Autodesk Inventor part; units mm, degrees
ref_plane "YZ Plane" through (0, 0, 0) normal (1, 0, 0) x (0, 1, 0)
ref_plane "XZ Plane" through (0, 0, 0) normal (0, 1, 0) x (-1, 0, 0)
ref_plane "XY Plane" through (0, 0, 0) normal (0, 0, 1) x (1, 0, 0)
sketch "スケッチ1" plane through (0, 0, 0) normal (0, 0, 1) x (1, 0, 0)
  line L0 (0, 0) -> (15, 0)
  line L1 (15, 0) -> (15, 30)
  line L2 (15, 30) -> (0, 30)
  line L3 (0, 30) -> (0, 0)
  line L4 (1, 1) -> (14, 1)
  line L5 (14, 1) -> (14, 29)
  line L6 (14, 29) -> (1, 29)
  line L7 (1, 29) -> (1, 1)
  dimension "d0" = 15
  dimension "d1" = 30
  dimension "d2" = 13
  dimension "d3" = 28
  dimension "d4" = 1
  dimension "d5" = 1
extrude "押し出し1" add sketch "スケッチ1" along normal blind 330
sketch "スケッチ2" plane through (0, 30, 0) normal (0, 1, 0) x (1, 0, 0)
  circle A0 centre (7.5, -15) radius 1.6
  line L0 (0, 0) -> (0, -330)
  line L1 (15, 0) -> (0, 0)
  circle A1 centre (7.5, -25) radius 1.6
  circle A2 centre (7.5, -35) radius 1.6
  circle A3 centre (7.5, -315) radius 1.6
  line L2 (15, -330) -> (0, -330)
  circle A4 centre (7.5, -305) radius 1.6
  circle A5 centre (7.5, -295) radius 1.6
  dimension "d8" = 3.2
  dimension "d9" = 7.5
  dimension "d10" = 15
  dimension "d11" = 3.2
  dimension "d12" = 10
  dimension "d13" = 3.2
  dimension "d14" = 10
  dimension "d15" = 3.2
  dimension "d16" = 15
  dimension "d17" = 7.5
  dimension "d18" = 3.2
  dimension "d19" = 10
  dimension "d20" = 3.2
  dimension "d21" = 10
hole "穴1" at (7.5, 30, 315) at (7.5, 30, 305) at (7.5, 30, 295) at (7.5, 30, 15) at (7.5, 30, 25) at (7.5, 30, 35) direction (0, -1, 0) diameter 3.2 depth 30
sketch "スケッチ3" plane through (0, 0, 0) normal (-1, 0, 0) x (0, 0, 1)
  circle A0 centre (10, 15) radius 1.6
  line L0 (0, 0) -> (330, 0)
  line L1 (0, 30) -> (0, 0)
  circle A1 centre (20, 15) radius 1.6
  circle A2 centre (30, 15) radius 1.6
  circle A3 centre (320, 15) radius 1.6
  line L2 (330, 30) -> (330, 0)
  circle A4 centre (310, 15) radius 1.6
  circle A5 centre (300, 15) radius 1.6
  dimension "d29" = 3.2
  dimension "d30" = 15
  dimension "d31" = 10
  dimension "d32" = 3.2
  dimension "d33" = 3.2
  dimension "d34" = 10
  dimension "d35" = 10
  dimension "d36" = 3.2
  dimension "d37" = 15
  dimension "d38" = 10
  dimension "d39" = 3.2
  dimension "d40" = 3.2
  dimension "d41" = 10
  dimension "d42" = 10
  dimension "d43" = 15
  dimension "d44" = 15
  dimension "d45" = 15
  dimension "d46" = 15
hole "穴2" at (0, 15, 10) at (0, 15, 20) at (0, 15, 30) at (0, 15, 300) at (0, 15, 310) at (0, 15, 320) direction (1, 0, 0) diameter 3.2 depth 15
sketch "スケッチ4" plane through (0, 0, 0) normal (-1, 0, 0) x (0, 0, 1)
  line L0 (165, 29.8281) -> (165, -0.1719) construction
  line L1 (0, 1) -> (330, 1)
  line L2 (165, 29.8281) -> (195, 29.8281) construction
  line L3 (0, 30) -> (0, 0)
  dimension "d54" = 30
  dimension "d55" = 90
  dimension "d56" = 165
sketch "スケッチ5" plane through (0, 0, 0) normal (-1, 0, 0) x (0, 0, 1)
  point P0 (0, 0)
sketch "スケッチ6" plane through (0, 0, 0) normal (-1, 0, 0) x (0, 0, 1)
  circle A0 centre (205.5, 23) radius 1.6
  circle A1 centre (205.5, 7) radius 1.6
  line L0 (0, 30) -> (330, 30)
  line L1 (0, 0) -> (330, 0)
  line L2 (0, 30) -> (0, 0)
  circle A2 centre (268.95, 23) radius 1.6
  circle A3 centre (268.95, 7) radius 1.6
  dimension "d57" = 3.2
  dimension "d58" = 3.2
  dimension "d59" = 16
  dimension "d60" = 7
  dimension "d61" = 7
  dimension "d62" = 205.5
  dimension "d63" = 3.2
  dimension "d64" = 63.45
  dimension "d65" = 7
  dimension "d66" = 3.2
  dimension "d67" = 16
  dimension "d68" = 7
hole "穴3" at (0, 23, 205.5) at (0, 7, 205.5) at (0, 23, 268.95) at (0, 7, 268.95) direction (1, 0, 0) diameter 3.2 depth 15
equation "\"BendRadius\" = Thickness"
equation "\"BendReliefWidth\" = Thickness"
equation "\"BendReliefDepth\" = 0.5 * Thickness"
equation "\"CornerReliefSize\" = 4 * Thickness"
equation "\"MinimumRemnant\" = 2 * Thickness"
equation "\"TransitionRadius\" = BendRadius"
equation "\"JacobiRadiusSize\" = BendRadius"
equation "\"GapSize\" = Thickness"
properties part number "nhk40"
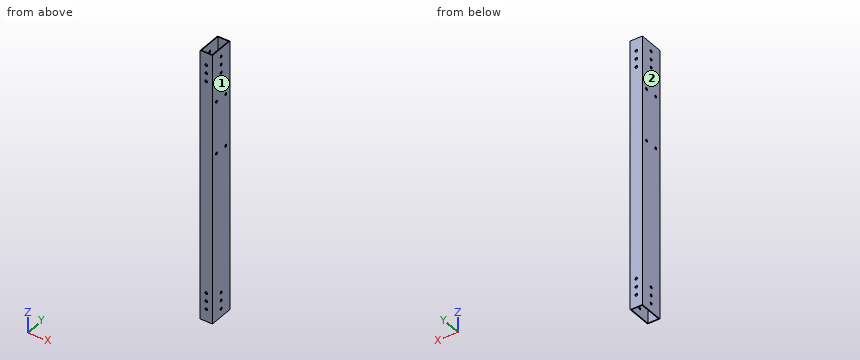
Design review of the part built by this model. Coordinates are the model's own, in mm. Face numbers are marked on the shaded views. Give positions to 0.01 mm unless a question says otherwise; leave off trailing zeros. Order: outer loops, then holes, each group sorted by start corner. A loop starts at its lowest first (then second) coordinate and runs counter-clockwise, first axis right, second up.
1. Mouldability with a two-part tool opening along X and no side actions: class the marked faces 1 and 2 as +X half, -X half, draft (parallel to the pull), parting line (faces both ways), or undercut.
Solution:
face 1: +X half
face 2: -X half
2. To check wall thickness, follow L1, parallel to Z at x = 0.65, y = 23; L2, parallel to Y at x = 0.3, z = 205.5; L3, parallel to X at y = 18.25, z = 217. State the ranges of each line that lie inside material, in increasing order.
Solution:
L1: z = 0 to 203.9, 207.1 to 267.35, 270.55 to 330
L2: y = 0 to 5.4, 8.6 to 21.4, 24.6 to 30
L3: x = 0 to 1, 14 to 15
3. Add section B-B, the plane x = 11.5. State the section outline as (y, z) points, then the cut area to 3 significant figures.
Solution:
outline: (0, 0) - (1, 0) - (1, 330) - (0, 330) - close; (29, 0) - (30, 0) - (30, 330) - (29, 330) - close
area: 660 mm2
4. Add section A-A, the plane z = 170.5. State the section outline as (x, y) points, then the cut area to 3 significant figures.
Solution:
outline: (0, 0) - (15, 0) - (15, 30) - (0, 30) - close; hole (1, 1) - (14, 1) - (14, 29) - (1, 29) - close
area: 86.0 mm2
